Work out the finished part from the listing and answer in its coordinate system (mm). Face numbers are marked on the shaded views. Coordinates: 2 decimals unless noted, no trailing zeros. Order: outer loops, then holes, each group sorted by start corner. A loop starts at its lowest first (then second) coordinate and runs counter-clockwise, first axis right, second up. Notation, with made-up numbers: M -6,83.25 L 22,83.25 A14 cw 22,102.25 Z; hole C 39.5,44.25 d10. An arc over 180 degrees is marked long. Answer in a Markdown table with one row per item. Add a question column.
Item 1: The part is cut by section D-D (y = 18). Write down the section's boundary in (x, z), then the cut area to 3 significant figures.
Item 2: The part is cut by section B-B (x = 0). Write down the section's boundary in (y, z), then the cut area to 3 significant figures.
Item 3: Flat-ended cylindrical pins translate along their axes: pin 1 Ø4.5 at (y, z) = (7, -0.5) entering from -X; pin 2 Ø3 at (x, z) = (45.5, -6.5) entering from +Y; pin 3 Ø12 at (y, z) = (8.5, 0) entering from +X; pin 4 Ø10 at (y, z) = (19.5, -4) entering from -X. Find the tip coordinate at first contact, or state that the pin passes through.
Item 4: Consider line 1 (Y direction, x = 0, z = 7.5); line 2 (Y direction, x = 0, z = 7.75); line 3 (Z direction, x = -32.5, y = 10). Determine where each line is inside the solid, lowest interval first. Write a range as from..to.
Item 5: The part is cut by section A-A (y = 8). Write down the section's boundary in (x, z).
Item 6: The mould has two halves that part along Z. Classify the marked faces 1, 2, 3 and 4: released by +Z, released by -Z, zero draft, split by the parting line, or undercut.
Item 7: The part is cut by section C-C (z = 2). Write down the section's boundary in (x, y), then the cut area to 3 significant figures.
Autodesk Inventor part; units mm, degrees
ref_plane "YZ Plane" through (0, 0, 0) normal (1, 0, 0) x (0, 1, 0)
ref_plane "XZ Plane" through (0, 0, 0) normal (0, 1, 0) x (-1, 0, 0)
ref_plane "XY Plane" through (0, 0, 0) normal (0, 0, 1) x (1, 0, 0)
sketch "Sketch1" plane through (0, 0, 0) normal (0, 1, 0) x (-1, 0, 0)
  line L0 (-9, 10.6795) -> (9, 10.6795)
  line L1 (9, 10.6795) -> (9, -4.7118)
  line L2 (9, -4.7118) -> (-9, -4.7118)
  line L3 (-9, -4.7118) -> (-9, 10.6795)
  line L4 (-9, 7.6795) -> (9, 7.6795)
  line L5 (-31.4348, -4.7118) -> (33.5217, -4.7118)
  line L6 (33.5217, -4.7118) -> (33.5217, -7.3205)
  line L7 (33.5217, -7.3205) -> (-31.4348, -7.3205)
  line L8 (-31.4348, -7.3205) -> (-31.4348, -4.7118)
  circle A0 centre (-43.3004, -6.0161) radius 5
  circle A1 centre (44.4458, -6.0161) radius 5
  point P0 (0, 0)
  point P1 (0, 7.6795)
  dimension "d6" = 3
  dimension "d7" = 18
  dimension "d8" = 18
  dimension "d34" = 10
  dimension "d35" = 10
extrude "Extrusion2" add sketch "Sketch1" along normal blind 3 contours L0 L1 L4 L3 | L4 L1 L2 L3 | L2 L5 L6 L7 L8
extrude "Extrusion3" add sketch "Sketch1" along normal blind 23 contours L0 L1 L4 L3
sketch "Sketch2" plane through (9, 3, 7.6795) normal (0, 0, -1) x (-1, 0, 0)
  line L0 (18, 0) -> (0, 0)
  line L1 (0, 20) -> (18, 20)
  circle A0 centre (9, 15) radius 2.25
  circle A1 centre (9, 5) radius 2.25
  circle A2 centre (9, 5) radius 4.25
  circle A3 centre (9, 15) radius 4.25
  point P0 (9, -3)
  point P1 (9, 20)
  point P2 (9, 0)
  dimension "d15" = 4.5
  dimension "d16" = 4.5
  dimension "d17" = 5
  dimension "d18" = 5
  dimension "d19" = 2
  dimension "d20" = 2
extrude "Extrusion4" cut sketch "Sketch2" against normal blind 3 contours A0 | A1
extrude "Extrusion5" add sketch "Sketch2" along normal blind 3
sketch "Sketch3" plane through (31.4348, 0, -7.3205) normal (0, 0, -1) x (-1, 0, 0)
  line L0 (64.9565, 0) -> (0, 0)
  line L1 (0, 3) -> (64.9565, 3)
  line L2 (24.4348, 23.1251) -> (38.4348, 23.1251)
  line L3 (38.4348, 23.1251) -> (38.4348, 3)
  line L4 (38.4348, 3) -> (24.4348, 3)
  line L5 (24.4348, 3) -> (24.4348, 23.1251)
  circle A0 centre (31.4348, 18) radius 2.25
  circle A1 centre (31.4348, 8) radius 2.25
  line L6 (0, 0) -> (0, 3)
  line L7 (-12.5217, -12.4797) -> (77.4783, -12.4797) construction
  arc A2 (77.4783, 0) -> (-12.5217, 0) centre (32.4783, -18.9639) ccw
  line L8 (-12.5217, 0) -> (77.4783, 0)
  point P0 (31.4348, 0)
  point P1 (32.4783, -12.4797)
  point P2 (32.4783, 0)
  dimension "d27" = 7
  dimension "d28" = 7
  dimension "d29" = 90
extrude "Extrusion6" add sketch "Sketch3" against normal blind 3 contours L0 L8 A2
fillet "Fillet1" radius 3 2 edges at (-46.0435, 0, -5.8205) (43.9565, 0, -5.8205)
fillet "Fillet2" radius 3 4 edges at (7, 3, -5.8205) (-7, 3, -5.8205) (-7, 23.1251, -5.8205) (7, 23.1251, -5.8205)
extrude "Extrusion8" add sketch "Sketch1" along normal blind 0.6 contours A0 | A1
properties part number "ZFoot"
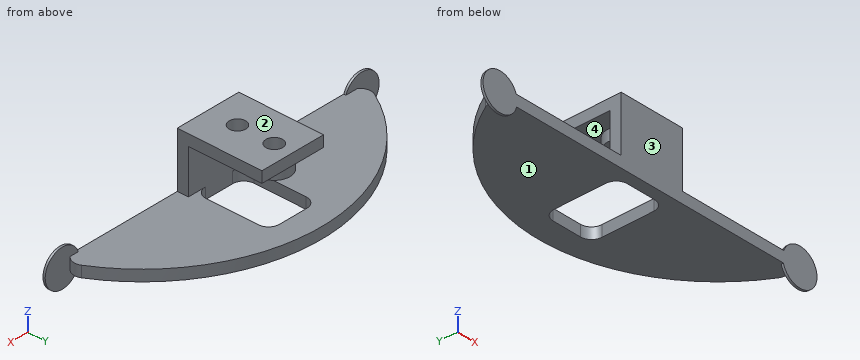
Reply:
| question | item | result |
|---|---|---|
| 1 | outline | M -32.95,-7.32 L -7,-7.32 L -7,-4.32 L -32.95,-4.32 Z; M -9,7.68 L -4.25,7.68 L -4.25,4.68 L -2.25,4.68 L -2.25,10.68 L -9,10.68 Z; M 2.25,4.68 L 4.25,4.68 L 4.25,7.68 L 9,7.68 L 9,10.68 L 2.25,10.68 Z; M 7,-7.32 L 30.87,-7.32 L 30.87,-4.32 L 7,-4.32 Z |
| 1 | area | 202 mm2 |
| 2 | outline | M 0,-7.32 L 3,-7.32 L 3,7.68 L 3.75,7.68 L 3.75,4.68 L 5.75,4.68 L 5.75,10.68 L 0,10.68 Z; M 10.25,4.68 L 12.25,4.68 L 12.25,7.68 L 13.75,7.68 L 13.75,4.68 L 15.75,4.68 L 15.75,10.68 L 10.25,10.68 Z; M 20.25,4.68 L 22.25,4.68 L 22.25,7.68 L 23,7.68 L 23,10.68 L 20.25,10.68 Z; M 23.13,-7.32 L 29.86,-7.32 L 29.86,-4.32 L 23.13,-4.32 Z |
| 2 | area | 131 mm2 |
| 3 | pin 1 | passes through |
| 3 | pin 2 | stops at y = 0.6 |
| 3 | pin 3 | stops at x = 41.87 |
| 3 | pin 4 | stops at x = -36.6 |
| 4 | line 1 | y = 0..3, 3.75..5.75, 10.25..12.25, 13.75..15.75, 20.25..22.25 |
| 4 | line 2 | y = 0..5.75, 10.25..15.75, 20.25..23 |
| 4 | line 3 | z = -7.32..-4.32 |
| 5 | outline | M -41.76,-7.32 L -7,-7.32 L -7,-4.32 L -41.76,-4.32 Z; M -9,7.68 L -4.25,7.68 L -4.25,4.68 L -2.25,4.68 L -2.25,10.68 L -9,10.68 Z; M 2.25,4.68 L 4.25,4.68 L 4.25,7.68 L 9,7.68 L 9,10.68 L 2.25,10.68 Z; M 7,-7.32 L 39.67,-7.32 L 39.67,-4.32 L 7,-4.32 Z |
| 6 | face 1 | released by -Z |
| 6 | face 2 | released by +Z |
| 6 | face 3 | zero draft |
| 6 | face 4 | undercut |
| 7 | outline | M -9,0 L 9,0 L 9,3 L -9,3 Z |
| 7 | area | 54.0 mm2 |
